Model file for the job. Use its own axes, mm. Round coordinates to 2 decimals unless told otherwise and drop trailing zeros. Loops run counter-clockwise (first coordinate to the right, second up) from the corner with the lowest first, then second, coordinate; pieces in that order, holes last. Notation, with made-up numbers: (36.25, 39) - (42.25, 39) arc R18 cw to (42.25, 71) - close; hole circle Ø8 at (-21, 41). An arc over 180 degrees is marked (long way). Answer as a JSON object with one key per item and string values.
from build123d import *

# Parameters (mm, degrees)
SKETCH_1_R      = 2.65
SKETCH_1_R_2    = 1.5
EXTRUDE_1_DEPTH = 90


with BuildPart() as part:
    # 草图1 → 凸台-拉伸1 (new, symmetric)
    with BuildSketch(Plane.XY):
        with BuildLine():
            Line((3.142893219, 3.85), (-3.142893219, 3.85))
            Line((-3.142893219, 3.85), (-5.5, 6.207106781))
            Line((-5.5, 6.207106781), (-5.5, 8.3))
            Line((-5.5, 8.3), (-3.1, 8.3))
            Line((-3.1, 8.3), (-3.1, 9.5))
            Line((-3.1, 9.5), (-3.6, 9.5))
            Line((-3.6, 9.5), (-3.6, 9.7))
            ThreePointArc((-3.6, 9.7), (-3.687867966, 9.912132034), (-3.9, 10))
            Line((-3.9, 10), (-8.5, 10))
            ThreePointArc((-8.5, 10), (-9.560660172, 9.560660172), (-10, 8.5))
            Line((-10, 8.5), (-10, 3.9))
            ThreePointArc((-10, 3.9), (-9.912132034, 3.687867966), (-9.7, 3.6))
            Line((-9.7, 3.6), (-9.5, 3.6))
            Line((-9.5, 3.6), (-9.5, 3.1))
            Line((-9.5, 3.1), (-8.3, 3.1))
            Line((-8.3, 3.1), (-8.3, 5.5))
            Line((-8.3, 5.5), (-6.207106781, 5.5))
            Line((-6.207106781, 5.5), (-3.85, 3.142893219))
            Line((-3.85, 3.142893219), (-3.85, -3.142893219))
            Line((-3.85, -3.142893219), (-6.207106781, -5.5))
            Line((-6.207106781, -5.5), (-8.3, -5.5))
            Line((-8.3, -5.5), (-8.3, -3.1))
            Line((-8.3, -3.1), (-9.5, -3.1))
            Line((-9.5, -3.1), (-9.5, -3.6))
            Line((-9.5, -3.6), (-9.7, -3.6))
            ThreePointArc((-9.7, -3.6), (-9.912132034, -3.687867966), (-10, -3.9))
            Line((-10, -3.9), (-10, -8.5))
            ThreePointArc((-10, -8.5), (-9.560660172, -9.560660172), (-8.5, -10))
            Line((-8.5, -10), (-3.9, -10))
            ThreePointArc((-3.9, -10), (-3.687867966, -9.912132034), (-3.6, -9.7))
            Line((-3.6, -9.7), (-3.6, -9.5))
            Line((-3.6, -9.5), (-3.1, -9.5))
            Line((-3.1, -9.5), (-3.1, -8.3))
            Line((-3.1, -8.3), (-5.5, -8.3))
            Line((-5.5, -8.3), (-5.5, -6.207106781))
            Line((-5.5, -6.207106781), (-3.142893219, -3.85))
            Line((-3.142893219, -3.85), (3.142893219, -3.85))
            Line((3.142893219, -3.85), (5.5, -6.207106781))
            Line((5.5, -6.207106781), (5.5, -8.3))
            Line((5.5, -8.3), (3.1, -8.3))
            Line((3.1, -8.3), (3.1, -9.5))
            Line((3.1, -9.5), (3.6, -9.5))
            Line((3.6, -9.5), (3.6, -9.7))
            ThreePointArc((3.6, -9.7), (3.687867966, -9.912132034), (3.9, -10))
            Line((3.9, -10), (8.5, -10))
            ThreePointArc((8.5, -10), (9.560660172, -9.560660172), (10, -8.5))
            Line((10, -8.5), (10, -3.9))
            ThreePointArc((10, -3.9), (9.912132034, -3.687867966), (9.7, -3.6))
            Line((9.7, -3.6), (9.5, -3.6))
            Line((9.5, -3.6), (9.5, -3.1))
            Line((9.5, -3.1), (8.3, -3.1))
            Line((8.3, -3.1), (8.3, -5.5))
            Line((8.3, -5.5), (6.207106781, -5.5))
            Line((6.207106781, -5.5), (3.85, -3.142893219))
            Line((3.85, -3.142893219), (3.85, 3.142893219))
            Line((3.85, 3.142893219), (6.207106781, 5.5))
            Line((6.207106781, 5.5), (8.3, 5.5))
            Line((8.3, 5.5), (8.3, 3.1))
            Line((8.3, 3.1), (9.5, 3.1))
            Line((9.5, 3.1), (9.5, 3.6))
            Line((9.5, 3.6), (9.7, 3.6))
            ThreePointArc((9.7, 3.6), (9.912132034, 3.687867966), (10, 3.9))
            Line((10, 3.9), (10, 8.5))
            ThreePointArc((10, 8.5), (9.560660172, 9.560660172), (8.5, 10))
            Line((8.5, 10), (3.9, 10))
            ThreePointArc((3.9, 10), (3.687867966, 9.912132034), (3.6, 9.7))
            Line((3.6, 9.7), (3.6, 9.5))
            Line((3.6, 9.5), (3.1, 9.5))
            Line((3.1, 9.5), (3.1, 8.3))
            Line((3.1, 8.3), (5.5, 8.3))
            Line((5.5, 8.3), (5.5, 6.207106781))
            Line((5.5, 6.207106781), (3.142893219, 3.85))
        make_face()
        with Locations(Location((0, 0, 0), (0, 0, 180))):
            Circle(SKETCH_1_R, mode=Mode.SUBTRACT)
        with Locations(Location((-7.75, 7.75, 0), (0, 0, 180))):
            Circle(SKETCH_1_R_2, mode=Mode.SUBTRACT)
        with Locations(Location((7.75, 7.75, 0), (0, 0, 180))):
            Circle(SKETCH_1_R_2, mode=Mode.SUBTRACT)
        with Locations(Location((7.75, -7.75, 0), (0, 0, 180))):
            Circle(SKETCH_1_R_2, mode=Mode.SUBTRACT)
        with Locations(Location((-7.75, -7.75, 0), (0, 0, 180))):
            Circle(SKETCH_1_R_2, mode=Mode.SUBTRACT)
    extrude(amount=EXTRUDE_1_DEPTH, both=True)


solid = part.part
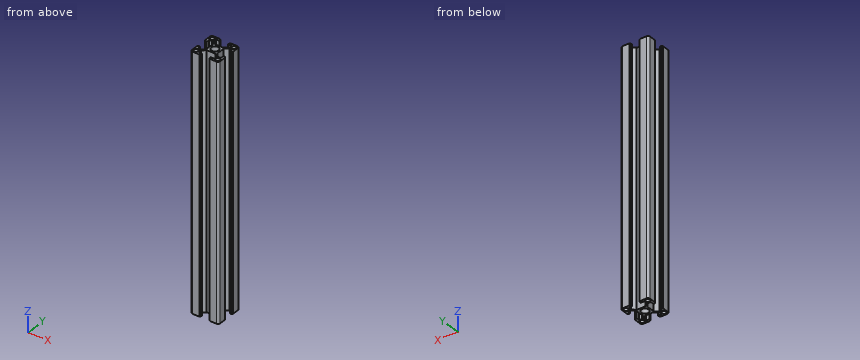
1) Slice it at C-C on z = -65. Count the separate pieces of the cut face and the enclosed holes in it, then the cut area to 3 significant figures.
Values follow:
{"separate pieces": "1", "enclosed holes": "5", "area": "130 mm²"}
2) Slice it at A-A on y = 0. List the corners of the cut face in (x, z), then the cut area to 3 significant figures.
Values follow:
{"outline": "(-3.85, -90) - (-2.65, -90) - (-2.65, 90) - (-3.85, 90) - close; (2.65, -90) - (3.85, -90) - (3.85, 90) - (2.65, 90) - close", "area": "432 mm²"}
3) Probe probe 1 along X at (y, z) = (7.75, 51.5); probe 2 along Y at (x, z) = (0, -5). List the from-to ranges inside material, lowest first.
Values follow:
{"probe 1": "-10 to -9.25, -6.25 to -5.5, 5.5 to 6.25, 9.25 to 10", "probe 2": "-3.85 to -2.65, 2.65 to 3.85"}
4) Drop flat-ended pins along their axis: P1, Ø0.6, axis at x = -9, z = 35.5, coming from the +Y side; P2, Ø0.6, axis at x = -3, z = 37.5, coming from the -Y side; P3, Ø0.6, axis at y = 9, z = -16.5, coming from the -X side. Give the stop position or say it passes through.
Values follow:
{"P1": "y = 9.99", "P2": "y = -9.5", "P3": "x = -9.99"}
